Model file for the job. Use its own axes, mm. Give positions to 0.01 mm unless a question says otherwise; leave off trailing zeros. Order: outer loops, then holes, each group sorted by start corner. A loop starts at its lowest first (then second) coordinate and runs counter-clockwise, first axis right, second up. Notation, with made-up numbers: (85.5, 65) - (140.5, 65) arc R26 cw to (140.5, 86) - close; hole circle Ø11 at (-11, 83.5). An arc over 180 degrees is marked (long way). Use CSV: the item, a comma, the result in double quotes. Start each with the question number.
(1) Band-saw the part on D-D, the plane z = 124. Give the cut face in (x, y), then the cut area to 3 significant figures.
(2) Band-saw the part on C-C, the plane z = 46.5. Give the cut face in (x, y), then the cut area to 3 significant figures.
(3) Band-saw the part on B-B, the plane y = -1298.5. Give the cut face in (x, z).
(4) Band-saw the part on A-A, the plane z = 212. Give the cut face in (x, y), then the cut area to 3 significant figures.
(5) Probe L1, parallel to Y at x = 10, z = 213.5; L2, parallel to X at y = -1172, z = 212; L3, parallel to X at y = -708, z = 74.5. List the from-to ranges inside material, lowest first.
(6) Drop flat-ended pins along their axis: pin 1 Ø12 at (y, z) = (-1030.5, 211) entering from +X; pin 2 Ø2 at (x, y) = (18.5, -750.5) entering from +Z; pin 3 Ø10 at (y, z) = (-1011.5, 34) entering from +X. Give the stop position or say it passes through.
from build123d import *

# Parameters (mm, degrees)
F0_R     = 250
F1_DEPTH = 2000
F3_W     = 886.840463
F3_H     = 523.860752
F4_DEPTH = 25
F6_DEPTH = 2000


with BuildPart() as f1:
    # F0 (on Front) → F1 (new body)
    with BuildSketch(Plane.XZ):
        Circle(F0_R)
    extrude(amount=F1_DEPTH)

    # F3 (on offset) → F4 (cut)
    with BuildSketch(Plane.XZ.offset(1500)):
        with Locations((77.082694, -5.228102)):
            Rectangle(F3_W, F3_H)
        with BuildLine():
            add(Edge.make_bspline(
                [(130, 0), (130, 311.769145), (-65, 155.884573), (-260, 0), (-65, -155.884573), (130, -311.769145), (130, 0)],
                knots=[4.712389, 4.712389, 4.712389, 6.806784, 6.806784, 8.901179, 8.901179, 10.995574, 10.995574, 10.995574], degree=2, weights=[1, 0.5, 1, 0.5, 1, 0.5, 1]))
        make_face(mode=Mode.SUBTRACT)
    extrude(amount=-F4_DEPTH, mode=Mode.SUBTRACT)

    # F5 (on face) → F6 (intersect)
    with BuildSketch(Plane.XZ.offset(2000)):
        with BuildLine():
            Line((0, 250), (0, 0))
            Line((0, 0), (21.788936, 249.048675))
            ThreePointArc((21.788936, 249.048675), (10.904847, 249.762055), (0, 250))
        make_face()
    extrude(amount=-F6_DEPTH, mode=Mode.INTERSECT)


solid = f1.part
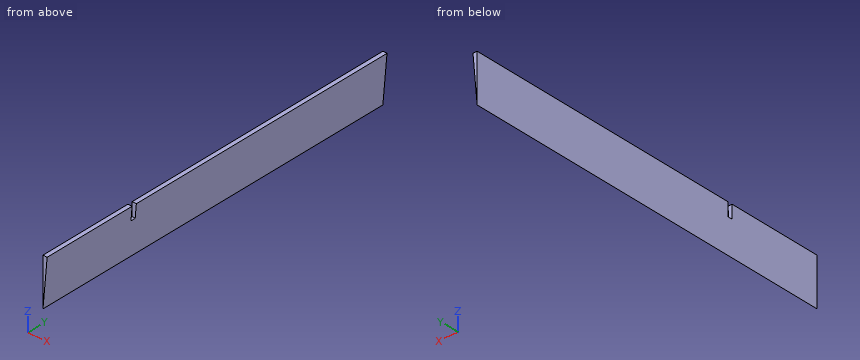
Answer block:
1,outline,"(0, -2000) - (10.85, -2000) - (10.85, 0) - (0, 0) - close"
1,area,"21,700 mm2"
2,outline,"(0, -2000) - (4.07, -2000) - (4.07, 0) - (0, 0) - close"
2,area,"8,140 mm2"
3,outline,"(0, 0) - (21.79, 249.05) arc R250 ccw to (0, 250) - close"
4,outline,"(0, -2000) - (18.55, -2000) - (18.55, -1500) - (0, -1500) - close; (0, -1475) - (18.55, -1475) - (18.55, 0) - (0, 0) - close"
4,area,"36,600 mm2"
5,L1,"y = -2000 to -1500, -1475 to 0"
5,L2,"x = 0 to 18.55"
5,L3,"x = 0 to 6.52"
6,pin 1,"stops at x = 18.99"
6,pin 2,"stops at z = 249.39"
6,pin 3,"stops at x = 3.41"
